Source: CAD feature listing. Evaluate the final solid. Frame: model axes, mm. A direction names the side the tool comes from. Round coordinates to 2 decimals unless told otherwise and drop trailing zeros. Order: outer loops, then holes, each group sorted by start corner. A loop starts at its lowest first (then second) coordinate and runs counter-clockwise, first axis right, second up. Notation, with made-up numbers: (36, 44.5) -> (87, 44.5) arc R25 cw to (87, 63.5) -> close; hole circle Ø1 at (70.5, 56.5). An arc over 180 degrees is marked (long way). One line per item, written item: value. Start each with the question number.
1) Section C-C (y = 8). Return the cut outline in (x, z).
2) Mould query, pull axis X, two halves, no side actions, for faces 4 (the face through (-0.73, 0.35, -0.16)), 5 (the face through (0.03, 1.42, -0.75)), 6 (the face through (1, 2, -2)). Classes: pulls with the +X half, pulls with the -X half, needs draft (parallel to the pull), parting line crosses it, or undercut.
3) Ray query, L1, parallel to X at y = 7, z = 0; L2, parallel to X at y = 6, z = 0; L3, parallel to Y at x = -3, z = 1.5. Return the intervals inside material, ascending.
4) Pin query (flat end, axial travel): P1, Ø4, axis at x = -1.5, y = 3, coming from the +Z side; P2, Ø1.5, axis at x = -1.5, y = 10.5, coming from the -Z side; P3, Ø1.2, axis at x = 0, z = 0, coming from the +Y side; P4, Ø2, axis at x = -2.5, z = 3, coming from the +Y side. Return the tip coordinate at first contact, or that it passes through.
5) Reachability of faces 1 (the face through (0, 9, -3)), 2 (the face through (-1.8, 3.5, -3)), 3 (the face through (0, 5, 3)) from +Z, -Z, +X, -X, +Y, -Y: full face, straight path, thin tool, end or side. Return the list, or none.
```python
from build123d import *

# Parameters (mm, degrees)
SKETCH_2_OUTSIDE_W  = 13.468
SKETCH_2_OUTSIDE_H  = 13.468
CUT_EXTRUDE_1_DEPTH = 3
CHAMFER_1_SIZE      = 0.6


with BuildPart() as part:
    # Эскиз1 → Повернуть1 (revolve)
    with BuildSketch(Plane(origin=(0, 0, 0), x_dir=(0, 0, -1), z_dir=(1, 0, 0))):
        Polygon((-0.4, 0.8), (-0.4, 0), (-0.5, 0), (-1.900415076, 2), (-4.04, 2), (-4.04, 5), (-2.5, 5), (-2.5, 6.5), (-3, 6.681985117), (-3, 12), (-2.5, 12.5), (-1, 12.5), (-1, 2), (-0.75, 1.849784845), (-0.75, 1.010301217), align=None)
    revolve(axis=Axis((0, 0, 0), (0, 1, 0)))

    # Эскиз2 outside → Вырез-Вытянуть1 (cut)
    with BuildSketch(Plane.XZ.offset(-2)):
        Rectangle(SKETCH_2_OUTSIDE_W, SKETCH_2_OUTSIDE_H)
        Polygon((0, 4.041451884), (-3.5, 2.020725942), (-3.5, -2.020725942), (0, -4.041451884), (3.5, -2.020725942), (3.5, 2.020725942), align=None, mode=Mode.SUBTRACT)
    extrude(amount=-CUT_EXTRUDE_1_DEPTH, mode=Mode.SUBTRACT)

    # Фаска1
    chamfer_1_edges = [part.edges().sort_by_distance(p)[0] for p in [
        (0, 12.5, -1),
    ]]
    chamfer(chamfer_1_edges, length=CHAMFER_1_SIZE)


solid = part.part
```
Findings:
1. outline: circle Ø6 at (0, 0); hole circle Ø2 at (0, 0)
2. face 4: parting line crosses it
2. face 5: undercut
2. face 6: needs draft
3. L1: -3 to -1, 1 to 3
3. L2: -2.5 to -1, 1 to 2.5
3. L3: 2 to 5
4. P1: z = 4.04
4. P2: z = -2.9
4. P3: y = 0.92
4. P4: y = 12.09
5. face 1: +Y
5. face 2: -Z, -X, +Y, -Y
5. face 3: none
